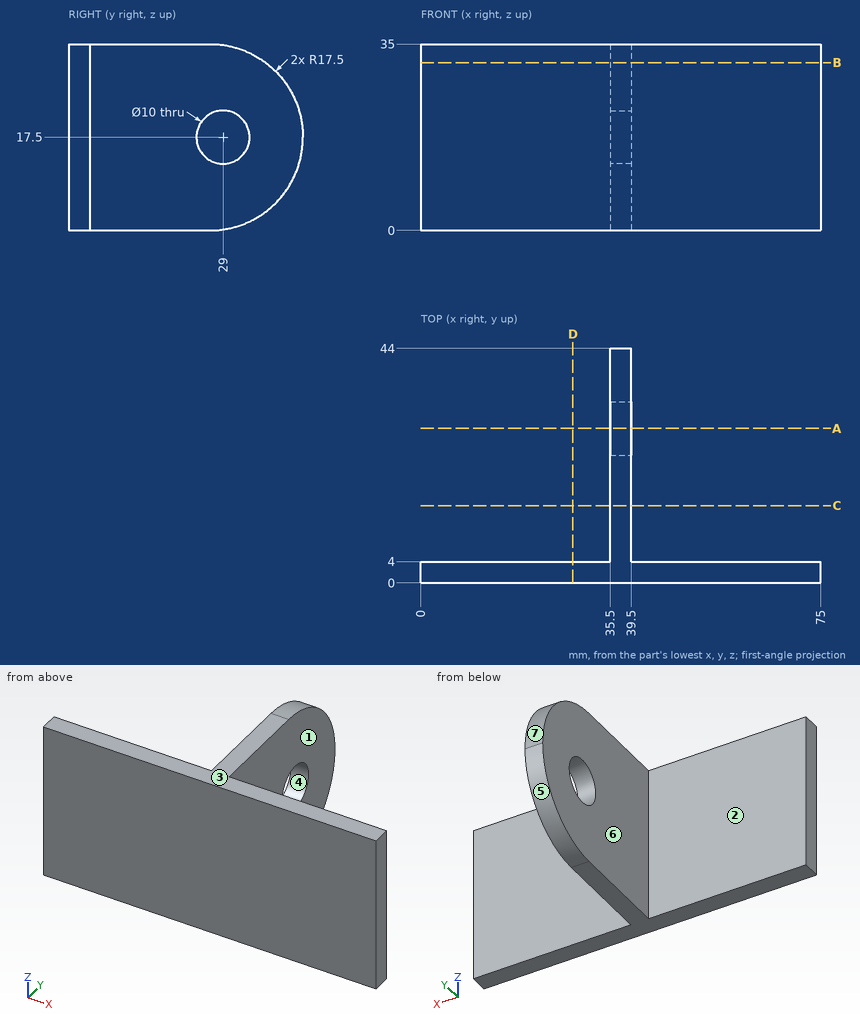
Could you check a few things on this drawing? It's one solid part, dimensions in mm from its lowest x, y, z. A direction names the side the tool comes from. Coordinates: 2 decimals unless noted, no trailing zeros. Order: outer loops, then holes, each group sorted by start corner. A loop starts at its lowest first (then second) coordinate and runs counter-clockwise, first axis right, second up. Notation, with made-up numbers: M 5.25,13.5 L 53.25,13.5 A25 cw 53.25,26.5 Z; hole C 13.25,80.5 d6. An arc over 180 degrees is marked long. Use a Markdown table: item, result. Add a question column.
Q1. If I drill on L1, parallel to Y at x = 36.5, z = 17.5; L2, parallel to Y at x = 42.5, z = 32; L3, parallel to X at y = 17, z = 20.5, over which ranges is the centre line in solid material (lowest first)?
Q2. I want a section at B-B on z = 31.5. List the corners of the cut face in (x, y) for me, then the cut area to 3 significant figures.
Q3. Which directions (+Z, -Z, +X, -X, +Y, -Y) give clear straight access to the entire face, cutting with the end or side of a thin tool? Please do the marked faces 1, 2 and 3.
Q4. We'd pull the mould along Z, two halves only. Please class the marked faces 4, 5, 6 and 7: pulls with the +Z half, pulls with the -Z half, needs draft (parallel to the pull), parting line crosses it, or undercut.
Q5. I want a section at D-D on x = 28.5. List the corners of the cut face in (y, z) for me, then the cut area to 3 significant figures.
Q6. I want a section at A-A on y = 29. List the corners of the cut face in (x, z) for me.
Q7. I want a section at C-C on y = 14.5. List the corners of the cut face in (x, z) for me, then the cut area to 3 significant figures.
Q8. I'm going to push flat-ended pins straight in: pin 1 (10.5 mm diameter, centred on y = 25, z = 19.5, fed in from -X); pin 2 (8 mm diameter, centred on y = 32, z = 29.5, fed in from +X); pin 3 (17.5 mm diameter, centred on x = 51, z = 12.5, fed in from +Y). Where does each tip first touch, or does it pass through?
Checked values:
| question | item | result |
|---|---|---|
| 1 | L1 | 0 to 24, 34 to 44 |
| 1 | L2 | 0 to 4 |
| 1 | L3 | 35.5 to 39.5 |
| 2 | outline | M 0,0 L 75,0 L 75,4 L 39.5,4 L 39.5,37 L 35.5,37 L 35.5,4 L 0,4 Z |
| 2 | area | 432 mm² |
| 3 | face 1 | +Z, -Z, +X, +Y |
| 3 | face 2 | +Z, -Z, -X, +Y |
| 3 | face 3 | +Z, +X, -X, +Y, -Y |
| 4 | face 4 | undercut |
| 4 | face 5 | pulls with the -Z half |
| 4 | face 6 | needs draft |
| 4 | face 7 | pulls with the +Z half |
| 5 | outline | M 0,0 L 4,0 L 4,35 L 0,35 Z |
| 5 | area | 140 mm² |
| 6 | outline | M 35.5,0.18 L 39.5,0.18 L 39.5,12.5 L 35.5,12.5 Z; M 35.5,22.5 L 39.5,22.5 L 39.5,34.82 L 35.5,34.82 Z |
| 7 | outline | M 35.5,0 L 39.5,0 L 39.5,35 L 35.5,35 Z |
| 7 | area | 140 mm² |
| 8 | pin 1 | x = 35.5 |
| 8 | pin 2 | x = 39.5 |
| 8 | pin 3 | y = 4 |
